Input: part model. Units: mm. Frame: model coordinates. A direction names the side the tool comes from. Coordinates: 2 decimals unless noted, no trailing zeros. Write each loop counter-clockwise with the first axis right and the second up, starting at its lowest first coordinate (ties: lowest second). Pieces come first, ordered by that corner, then holes. Notation, with made-up numbers: (36.5, -31.75) - (52.5, -31.75) arc R22 cw to (52.5, -20.75) - close; hole circle Ø10 at (31, -29). An arc over 180 degrees is marked (long way). Put each result on its own line as item: value. Start each with the question number.
1. Cut plane C-C, the plane y = 16.5. Return loops of the section in (x, z), and give its area (3 significant figures).
2. Cut plane A-A, the plane z = 4. Return loops of the section in (x, y) (3 decimals), and give its area (3 significant figures).
3. Pin query (flat end, axial travel): pin 1 (6 mm diameter, centred on y = -24, z = 1.5, fed in from +X); pin 2 (8 mm diameter, centred on x = -16, z = 1, fed in from +Y); pin 3 (5 mm diameter, centred on x = -8.99, y = 49.19, fed in from +Z); pin 4 (2 mm diameter, centred on y = -12, z = 14.5, fed in from +X). Return the tip coordinate at first contact, or that it passes through.
4. Pull-direction query (X, two-part tool) for faces 1 (the flat face through (-1, 1, -3)), 2 (the flat face through (-1, 1, 0)), 3 (the cylindrical face through (-11.923, -53.692, 9.675)); classes: released by +X, released by -X, zero draft, split by the parting line, or undercut.
5. Line query: line 1 (X direction, y = -17, z = 12.5); line 2 (Y direction, x = 0, z = 9.75); line 3 (Y direction, x = -11, z = 18.25). Output: solid intervals per line, ascending.
6. Access query for faces 4 (the cylindrical face through (20.765, -39.923, 10.846)), 5 (the cylindrical face through (-7.07, 50.36, 9.32)). Directions: +Z, -Z, +X, -X, +Y, -Y. A direction counts if a zero-diameter tool reaches every point of the face in a straight line with its end or side. Return the directions, or none.
7. Cut plane B-B, the plane x = 0. Return loops of the section in (y, z).
from build123d import *

# Parameters (mm, degrees)
F0_R     = 55
F0_R_2   = 45
F1_DEPTH = 22
F2_DEPTH = 3


with BuildPart() as f1:
    # F0 (on Top) → F1 (new body)
    with BuildSketch(Plane.XY):
        Circle(F0_R)
        with BuildLine():
            ThreePointArc((-6.7686770228, 49.539731644), (32.8752653895, 37.6724956111), (50, 0))
            ThreePointArc((50, 0), (49.4467404253, -7.417537416), (47.7992055473, -14.6709218881))
            ThreePointArc((47.7992055473, -14.6709218881), (48.9151264842, -15.489568044), (49.3407844988, -16.8064872976))
            ThreePointArc((49.3407844988, -16.8064872976), (48.3663226704, -18.6599981211), (46.2870046118, -18.9080195703))
            ThreePointArc((46.2870046118, -18.9080195703), (8.9905473014, -49.1850593089), (-36.6049938257, -34.0598653406))
            ThreePointArc((-36.6049938257, -34.0598653406), (-39.8147478714, -33.8356077519), (-39.518327589, -30.6317120738))
            ThreePointArc((-39.518327589, -30.6317120738), (-47.0907844988, 16.8064872976), (-11.1942117216, 48.7307872287))
            ThreePointArc((-11.1942117216, 48.7307872287), (-9.3951219299, 51.3983869778), (-6.7686770228, 49.539731644))
        make_face(mode=Mode.SUBTRACT)
        with BuildLine():
            ThreePointArc((47.7992055473, -14.6709218881), (49.4467404253, -7.417537416), (50, 0))
            ThreePointArc((50, 0), (32.8752653895, 37.6724956111), (-6.7686770228, 49.539731644))
            ThreePointArc((-6.7686770228, 49.539731644), (-6.7475907562, 49.3629523572), (-6.7405473014, 49.1850593089))
            ThreePointArc((-6.7405473014, 49.1850593089), (-8.7622327657, 46.9466731776), (-11.1942117216, 48.7307872287))
            ThreePointArc((-11.1942117216, 48.7307872287), (-47.0907844988, 16.8064872976), (-39.518327589, -30.6317120738))
            ThreePointArc((-39.518327589, -30.6317120738), (-37.1328188239, -30.3471681395), (-35.8502371975, -32.3785720114))
            ThreePointArc((-35.8502371975, -32.3785720114), (-36.0475806765, -33.3000388891), (-36.6049938257, -34.0598653406))
            ThreePointArc((-36.6049938257, -34.0598653406), (8.9905473014, -49.1850593089), (46.2870046118, -18.9080195703))
            ThreePointArc((46.2870046118, -18.9080195703), (44.9716991964, -16.0501953692), (47.7992055473, -14.6709218881))
        make_face()
        Circle(F0_R_2, mode=Mode.SUBTRACT)
    extrude(amount=F1_DEPTH)

    # F0 (on Top) → F2 (join)
    with BuildSketch(Plane.XY):
        Circle(F0_R)
        with BuildLine():
            ThreePointArc((-6.7686770228, 49.539731644), (32.8752653895, 37.6724956111), (50, 0))
            ThreePointArc((50, 0), (49.4467404253, -7.417537416), (47.7992055473, -14.6709218881))
            ThreePointArc((47.7992055473, -14.6709218881), (48.9151264842, -15.489568044), (49.3407844988, -16.8064872976))
            ThreePointArc((49.3407844988, -16.8064872976), (48.3663226704, -18.6599981211), (46.2870046118, -18.9080195703))
            ThreePointArc((46.2870046118, -18.9080195703), (8.9905473014, -49.1850593089), (-36.6049938257, -34.0598653406))
            ThreePointArc((-36.6049938257, -34.0598653406), (-39.8147478714, -33.8356077519), (-39.518327589, -30.6317120738))
            ThreePointArc((-39.518327589, -30.6317120738), (-47.0907844988, 16.8064872976), (-11.1942117216, 48.7307872287))
            ThreePointArc((-11.1942117216, 48.7307872287), (-9.3951219299, 51.3983869778), (-6.7686770228, 49.539731644))
        make_face(mode=Mode.SUBTRACT)
        with BuildLine():
            ThreePointArc((47.7992055473, -14.6709218881), (49.4467404253, -7.417537416), (50, 0))
            ThreePointArc((50, 0), (32.8752653895, 37.6724956111), (-6.7686770228, 49.539731644))
            ThreePointArc((-6.7686770228, 49.539731644), (-6.7475907562, 49.3629523572), (-6.7405473014, 49.1850593089))
            ThreePointArc((-6.7405473014, 49.1850593089), (-8.7622327657, 46.9466731776), (-11.1942117216, 48.7307872287))
            ThreePointArc((-11.1942117216, 48.7307872287), (-47.0907844988, 16.8064872976), (-39.518327589, -30.6317120738))
            ThreePointArc((-39.518327589, -30.6317120738), (-37.1328188239, -30.3471681395), (-35.8502371975, -32.3785720114))
            ThreePointArc((-35.8502371975, -32.3785720114), (-36.0475806765, -33.3000388891), (-36.6049938257, -34.0598653406))
            ThreePointArc((-36.6049938257, -34.0598653406), (8.9905473014, -49.1850593089), (46.2870046118, -18.9080195703))
            ThreePointArc((46.2870046118, -18.9080195703), (44.9716991964, -16.0501953692), (47.7992055473, -14.6709218881))
        make_face()
        Circle(F0_R_2, mode=Mode.SUBTRACT)
        Circle(F0_R_2)
    extrude(amount=-F2_DEPTH)


solid = f1.part
Report:
1. outline: (-52.47, -3) - (52.47, -3) - (52.47, 22) - (41.87, 22) - (41.87, 0) - (-41.87, 0) - (-41.87, 22) - (-52.47, 22) - close
1. area: 781 mm^2
2. outline: circle Ø110 at (0, 0); hole circle Ø90 at (0, 0); hole circle Ø4.5 at (-38.1, -32.379); hole circle Ø4.5 at (-8.991, 49.185); hole circle Ø4.5 at (47.091, -16.806)
2. area: 3,090 mm^2
3. pin 1: stops at x = 50.83
3. pin 2: stops at y = 53.67
3. pin 3: stops at z = 22
3. pin 4: stops at x = 53.89
4. face 1: zero draft
4. face 2: undercut
4. face 3: split by the parting line
5. line 1: x = -52.31 to -41.67, 41.67 to 44.85, 49.33 to 52.31
5. line 2: y = -55 to -45, 45 to 55
5. line 3: y = -53.89 to -43.63, 43.63 to 48.17, 50.2 to 53.89
6. face 4: +Z
6. face 5: +Z, -Z
7. outline: (-55, -3) - (55, -3) - (55, 22) - (45, 22) - (45, 0) - (-45, 0) - (-45, 22) - (-55, 22) - close
